Input: part model. Units: mm. Frame: model coordinates. A direction names the side the tool comes from. Give positions to 0.01 mm unless a question says otherwise; leave off trailing zeros. Loops run counter-clockwise (first coordinate to the right, second up) from the corner with the lowest first, then second, coordinate; pieces in that order, holes last. Notation, with made-up numbers: (74.5, 71) - (91.5, 71) arc R17 cw to (91.5, 93) - close; hole circle Ø5 at (-24.5, -12.5). An arc over 180 degrees is marked (long way). Answer as a JSON object with one key per item and string values. Group by question number.
(1) Access query for faces 4 (the cylindrical face through (19, 30.8, 5.1)), 5 (the flat face through (3, 11, -7)), 6 (the flat face through (24, 11, 5)), 7 (the flat face through (27, 19, 5)). Directions: +Z, -Z, +X, -X, +Y, -Y. A direction counts if a zero-diameter tool reaches every point of the face in a straight line with its end or side. Return the directions, or none.
(2) Section query B-B (x = 2). Return loops of the section in (y, z).
(3) Section query C-C (z = 5.5). Return loops of the section in (x, y), plus the area to 3 significant figures.
(4) Section query D-D (y = 10). Return loops of the section in (x, z), plus the area to 3 significant figures.
(5) Mould query, pull axis Y, two halves, no side actions, for faces 1 (the cylindrical face through (11, 19, 13)), 2 (the flat face through (24, 27, 5)), 3 (the cylindrical face through (35.46, 35.16, 0.79)). Classes: +Y half, -Y half, draft (parallel to the pull), parting line (faces both ways), or undercut.
(6) Pin query (flat end, axial travel): P1, Ø2, axis at x = 26, z = -0.5, coming from the +Y side; P2, Ø1, axis at y = 10, z = 4.5, coming from the -X side; P3, Ø3.5, axis at y = 20, z = 5, coming from the -X side; P4, Ø2, axis at x = 17, z = 5.5, coming from the +Y side. Return the tip coordinate at first contact, or that it passes through.
(7) Section query A-A (y = 36). Return loops of the section in (x, z), plus the area to 3 significant figures.
(8) Material intervals for L1, parallel to Y at x = 2, z = 1; L2, parallel to Z at x = 8, y = 29.5; L3, parallel to Y at x = 2, z = -3.5, sorted ascending.
```python
from build123d import *

# Parameters (mm, degrees)
ESQUISSE1_W        = 38
ESQUISSE1_H        = 38
ESQUISSE1_R        = 1
BOSS_EXTRU_1_DEPTH = 1.6
BOSS_EXTRU_2_DEPTH = 7
ESQUISSE3_R        = 8
BOSS_EXTRU_3_DEPTH = 10
CHANFREIN1_SIZE    = 1
CHANFREIN1_SIZE2   = 1.732050808
CONG_1_R           = 10
ESQUISSE4_W        = 6
ESQUISSE4_H        = 10
BOSS_EXTRU_4_DEPTH = 14


with BuildPart() as part:
    # Esquisse1 → Boss.-Extru.1 (new body)
    with BuildSketch(Plane.XY):
        with Locations((19, 19)):
            Rectangle(ESQUISSE1_W, ESQUISSE1_H)
        with Locations((2, 36)):
            Circle(ESQUISSE1_R, mode=Mode.SUBTRACT)
        with Locations((2, 2)):
            Circle(ESQUISSE1_R, mode=Mode.SUBTRACT)
        with Locations(Location((36, 2, 0), (0, 0, 180))):
            Circle(ESQUISSE1_R, mode=Mode.SUBTRACT)
        with Locations(Location((36, 36, 0), (0, 0, 180))):
            Circle(ESQUISSE1_R, mode=Mode.SUBTRACT)
    extrude(amount=BOSS_EXTRU_1_DEPTH)

    # Esquisse2 → Boss.-Extru.2 (add)
    with BuildSketch(Plane.XY.offset(1.6)):
        with BuildLine():
            Line((11, 27), (17.2, 27))
            Line((17.2, 27), (17.2, 29))
            ThreePointArc((17.2, 29), (19, 30.8), (20.8, 29))
            Line((20.8, 29), (20.8, 27))
            Line((20.8, 27), (27, 27))
            Line((27, 27), (27, 11))
            Line((27, 11), (20.8, 11))
            Line((20.8, 11), (20.8, 9))
            ThreePointArc((20.8, 9), (19, 7.2), (17.2, 9))
            Line((17.2, 9), (17.2, 11))
            Line((17.2, 11), (11, 11))
            Line((11, 11), (11, 27))
        make_face()
    extrude(amount=BOSS_EXTRU_2_DEPTH)

    # Esquisse3 → Boss.-Extru.3 (add)
    with BuildSketch(Plane.XY.offset(8.6)):
        with Locations((19, 19)):
            Circle(ESQUISSE3_R)
    extrude(amount=BOSS_EXTRU_3_DEPTH)

    # Chanfrein1
    chanfrein1_edges = [part.edges().sort_by_distance(p)[0] for p in [
        (11, 19, 18.6),
    ]]
    chanfrein1_side = [part.faces().sort_by_distance(p)[0] for p in [
        (11, 19, 13.6),
    ]]
    chamfer(chanfrein1_edges, length=CHANFREIN1_SIZE, length2=CHANFREIN1_SIZE2, reference=chanfrein1_side[0])

    # Congé1
    # the kernel refuses this fillet: 10 mm, written as the material it takes off along each edge
    with BuildSketch(Plane(origin=(19, 19, 18.6), x_dir=(1, 0, 0), z_dir=(0, -1, 0))) as cong_1_piece_1:
        with BuildLine():
            CenterArc((3.641101056, -10), CONG_1_R, 64.158067237, 25.841932763)
            Line((3.641101056, 0), (3.641101056, 0.2))
            Line((3.641101056, 0.2), (6.267949192, 0.2))
            Line((6.267949192, 0.2), (6.367949192, 0.173205081))
            ThreePointArc((6.367949192, 0.173205081), (7.233974596, -0.326794919), (8.087177979, -0.82))
            Line((8.087177979, -0.82), (8, -1))
        make_face()
    revolve(axis=Axis((19, 19, 18.6), (0, 0, 1)), mode=Mode.SUBTRACT)

    # Esquisse4 → Boss.-Extru.4 (add)
    with BuildSketch(Plane(origin=(0, 0, 0), x_dir=(-1, 0, 0), z_dir=(0, 0, -1))):
        with Locations((-3, 16)):
            Rectangle(ESQUISSE4_W, ESQUISSE4_H)
    extrude(amount=BOSS_EXTRU_4_DEPTH)


solid = part.part
```
Recorded:
{
 "1": {"face 4": "+Z, +Y", "face 5": "-Z, +X, -X, -Y", "face 6": "+Z, +X, -Y", "face 7": "+Z, +X, +Y, -Y"},
 "2": {"outline": "(0, 0) - (1, 0) - (1, 1.6) - (0, 1.6) - close; (3, 0) - (11, 0) - (11, -14) - (21, -14) - (21, 0) - (35, 0) - (35, 1.6) - (3, 1.6) - close; (37, 0) - (38, 0) - (38, 1.6) - (37, 1.6) - close"},
 "3": {"outline": "(11, 11) - (17.2, 11) - (17.2, 9) arc R1.8 ccw to (20.8, 9) - (20.8, 11) - (27, 11) - (27, 27) - (20.8, 27) - (20.8, 29) arc R1.8 ccw to (17.2, 29) - (17.2, 27) - (11, 27) - close", "area": "281 mm^2"},
 "4": {"outline": "(0, 0) - (38, 0) - (38, 1.6) - (20.8, 1.6) - (20.8, 8.6) - (17.2, 8.6) - (17.2, 1.6) - (0, 1.6) - close", "area": "86.0 mm^2"},
 "5": {"face 1": "parting line", "face 2": "+Y half", "face 3": "undercut"},
 "6": {"P1": "stops at y = 38", "P2": "stops at x = 17.2", "P3": "stops at x = 11", "P4": "stops at y = 30.5"},
 "7": {"outline": "(0, 0) - (1, 0) - (1, 1.6) - (0, 1.6) - close; (3, 0) - (35, 0) - (35, 1.6) - (3, 1.6) - close; (37, 0) - (38, 0) - (38, 1.6) - (37, 1.6) - close", "area": "54.4 mm^2"},
 "8": {"L1": "y = 0 to 1, 3 to 35, 37 to 38", "L2": "z = 0 to 1.6", "L3": "y = 11 to 21"}
}
